Read the model definition and answer for the solid it produces. Units are mm, in the model's axes. A direction names the side the tool comes from. Coordinates: 2 decimals unless noted, no trailing zeros. Order: outer loops, then holes, each group sorted by start corner. A loop starts at its lowest first (then second) coordinate and runs counter-clockwise, first axis right, second up. Notation, with made-up numbers: (83, -18.5) -> (120, -18.5) arc R9 cw to (120, -5.5) -> close; hole circle Ø6 at (-4, -10). An arc over 180 degrees is marked (long way). Use CSV: the item, a comma, the result in double quotes.
```python
from build123d import *

# Parameters (mm, degrees)
SZKIC1_W                    = 1.6
SZKIC1_H                    = 10.8
DODANIE_WYCI_GNI_CIE1_DEPTH = 60
SZKIC2_R                    = 1.25
WYTNIJ_WYCI_GNI_CIE1_DEPTH  = 60
SZKIC3_W                    = 1.6
SZKIC3_H                    = 2
WYTNIJ_WYCI_GNI_CIE2_DEPTH  = 2.6
SZKIC4_W                    = 1.6
SZKIC4_H                    = 2
DODANIE_WYCI_GNI_CIE2_DEPTH = 3
WYTNIJ_WYCI_GNI_CIE3_START  = -30.75
SZKIC6_W                    = 1.6
SZKIC6_H                    = 3
SZKIC6_H_2                  = 3.1
WYTNIJ_WYCI_GNI_CIE3_DEPTH  = 30.75
SZKIC7_W                    = 1.6
SZKIC7_H                    = 4.7
WYTNIJ_WYCI_GNI_CIE4_DEPTH  = 9.35
SZKIC8_W                    = 1.6
SZKIC8_H                    = 1.6
DODANIE_WYCI_GNI_CIE3_DEPTH = 3
SZKIC9_R                    = 0.375
SZKIC9_R_2                  = 0.37655367
SZKIC9_R_3                  = 0.375938448
WYTNIJ_WYCI_GNI_CIE5_DEPTH  = 1.6


with BuildPart() as part:
    # Szkic1 → Dodanie-wyciągnięcie1 (new body)
    with BuildSketch(Plane.XY):
        with Locations((-22.216876634, 9.987687188)):
            Rectangle(SZKIC1_W, SZKIC1_H)
    extrude(amount=DODANIE_WYCI_GNI_CIE1_DEPTH)

    # Szkic2 → Wytnij-wyciągnięcie1 (cut)
    with BuildSketch(Plane(origin=(-21.416876634, 0, 0), x_dir=(0, 0, -1), z_dir=(1, 0, 0))):
        with Locations((-56.5, 9.987687188)):
            Circle(SZKIC2_R)
        with Locations((-48.5, 9.987687188)):
            Circle(SZKIC2_R)
    extrude(amount=-WYTNIJ_WYCI_GNI_CIE1_DEPTH, mode=Mode.SUBTRACT)

    # Szkic3 → Wytnij-wyciągnięcie2 (cut)
    with BuildSketch(Plane(origin=(0, 15.387687188, 0), x_dir=(1, 0, 0), z_dir=(0, 1, 0))):
        with Locations((-22.216876634, -37.6)):
            Rectangle(SZKIC3_W, SZKIC3_H)
    extrude(amount=-WYTNIJ_WYCI_GNI_CIE2_DEPTH, mode=Mode.SUBTRACT)

    # Szkic4 → Dodanie-wyciągnięcie2 (add)
    with BuildSketch(Plane.XZ.offset(-4.587687188)):
        with Locations((-22.216876634, 39.6)):
            Rectangle(SZKIC4_W, SZKIC4_H)
    extrude(amount=DODANIE_WYCI_GNI_CIE2_DEPTH)

    # Szkic6 → Wytnij-wyciągnięcie3 (cut)
    with BuildSketch(Plane(origin=(0, 0, 0), x_dir=(-1, 0, 0), z_dir=(0, 0, -1)).offset(WYTNIJ_WYCI_GNI_CIE3_START)):
        with Locations((22.216876634, 13.887687188)):
            Rectangle(SZKIC6_W, SZKIC6_H)
        with Locations((22.216876634, 6.137687188)):
            Rectangle(SZKIC6_W, SZKIC6_H_2)
    extrude(amount=WYTNIJ_WYCI_GNI_CIE3_DEPTH, mode=Mode.SUBTRACT)

    # Szkic7 → Wytnij-wyciągnięcie4 (cut)
    with BuildSketch(Plane(origin=(0, 0, 0), x_dir=(-1, 0, 0), z_dir=(0, 0, -1))):
        with Locations((22.216876634, 10.037687188)):
            Rectangle(SZKIC7_W, SZKIC7_H)
    extrude(amount=-WYTNIJ_WYCI_GNI_CIE4_DEPTH, mode=Mode.SUBTRACT)

    # Szkic8 → Dodanie-wyciągnięcie3 (add)
    with BuildSketch(Plane.XZ.offset(-4.587687188)):
        with Locations((-22.216876634, 37.8)):
            Rectangle(SZKIC8_W, SZKIC8_H)
    extrude(amount=DODANIE_WYCI_GNI_CIE3_DEPTH)

    # Szkic9 → Wytnij-wyciągnięcie5 (cut)
    with BuildSketch(Plane.ZY.offset(23.016876634)):
        with Locations((37, 4.212687188)):
            Circle(SZKIC9_R)
        with Locations((38.565828862, 13.162687188)):
            Circle(SZKIC9_R_2)
        with Locations((36.573453505, 13.162687188)):
            Circle(SZKIC9_R_3)
    extrude(amount=-WYTNIJ_WYCI_GNI_CIE5_DEPTH, mode=Mode.SUBTRACT)


solid = part.part
```
Item 1: A tool of negligible diameter and unlimited length cuts with its end or side. For faces 4 (the flat face through (-22, 14, 38.6)), 5 (the flat face through (-22, 4.588, 50)), 6 (the flat face through (-22, 7.688, 20)), from which of +Z, -Z, +X, -X, +Y, -Y can it reach the whole face along a straight path? Write none if from no direction.
Return value:
face 4,"+X, -X, +Y"
face 5,"+Z, +X, -X, -Y"
face 6,"-Z, +X, -X, -Y"
Item 2: The mould has two halves that part along Z. Classify faces 1 (the flat face through (-22, 14, 30.75)), 2 (the flat face through (-22, 12.388, 20)), 3 (the flat face through (-22, 12.788, 38)): +Z half, -Z half, draft (parallel to the pull), parting line (faces both ways), or undercut.
Return value:
face 1,"-Z half"
face 2,"draft"
face 3,"undercut"
Item 3: Each of these flat-tipped pins is pushed along its axis until it touches: P1, Ø0.8, axis at x = -22, z = 54, coming from the -Y side; P2, Ø0.8, axis at x = -22.5, y = 3, coming from the -Z side; P3, Ø0.5, axis at x = -22, z = 17.5, coming from the +Y side. Where does it stop, or does it pass through?
Return value:
P1,"stops at y = 4.59"
P2,"stops at z = 37"
P3,"stops at y = 12.39"
Item 4: Straight lines are drawn through the part: line 1 along Y through (x, z) = (-21.85, 48.5); line 2 along Z through (x, y) = (-21.9, 10.25); line 3 along Z through (x, y) = (-22.55, 13.75). For each, find the intervals that lie inside material, in ascending order.
Return value:
line 1,"y = 4.59 to 8.74, 11.24 to 15.39"
line 2,"z = 9.35 to 47.28, 49.72 to 55.28, 57.72 to 60"
line 3,"z = 30.75 to 36.6, 38.6 to 60"
Item 5: Find section D-D, the plane z = 28. Give the vertices of the cut face in (x, y), then the cut area to 3 significant figures.
Return value:
outline,"(-23.02, 7.69) -> (-21.42, 7.69) -> (-21.42, 12.39) -> (-23.02, 12.39) -> close"
area,"7.52 mm^2"
Item 6: Find section C-C, the plane x = -22.75. Give the vertices of the cut face in (y, z) (3 decimals), then the cut area to 3 significant figures.
Return value:
outline,"(1.588, 37) -> (3.838, 37) arc R0.375 cw to (4.588, 37) -> (4.588, 30.75) -> (7.688, 30.75) -> (7.688, 9.35) -> (12.388, 9.35) -> (12.388, 30.75) -> (15.388, 30.75) -> (15.388, 36.6) -> (13.538, 36.6) arc R0.376 cw (long way) to (12.788, 36.6) -> (12.788, 38.532) arc R0.377 cw to (13.538, 38.6) -> (15.388, 38.6) -> (15.388, 60) -> (4.588, 60) -> (4.588, 40.6) -> (1.588, 40.6) -> close; hole circle Ø2.5 at (9.988, 48.5); hole circle Ø2.5 at (9.988, 56.5)"
area,"412 mm^2"
Item 7: Find section A-A, the plane z = 48.5. Give the vertices of the cut face in (x, y), then the cut area to 3 significant figures.
Return value:
outline,"(-23.02, 4.59) -> (-21.42, 4.59) -> (-21.42, 8.74) -> (-23.02, 8.74) -> close; (-23.02, 11.24) -> (-21.42, 11.24) -> (-21.42, 15.39) -> (-23.02, 15.39) -> close"
area,"13.3 mm^2"
Item 8: Find section B-B, the plane y = 10.75. Give the vertices of the cut face in (x, z), then the cut area to 3 significant figures.
Return value:
outline,"(-23.02, 9.35) -> (-21.42, 9.35) -> (-21.42, 47.51) -> (-23.02, 47.51) -> close; (-23.02, 49.49) -> (-21.42, 49.49) -> (-21.42, 55.51) -> (-23.02, 55.51) -> close; (-23.02, 57.49) -> (-21.42, 57.49) -> (-21.42, 60) -> (-23.02, 60) -> close"
area,"74.7 mm^2"
